Input: part model. Units: mm. Frame: model coordinates. Face numbers are marked on the shaded views. A direction names the side the tool comes from. Round coordinates to 2 decimals unless told otherwise and drop trailing zeros. Loops run counter-clockwise (first coordinate to the right, second up) from the corner with the lowest first, then second, coordinate; pieces in that order, holes last. Notation, with made-up numbers: (-21.5, 86.5) - (31.5, 86.5) arc R23 ccw to (31.5, 96.5) - close; hole circle Ø7 at (23, -26). An arc over 180 degrees is marked (long way). One line per question, with ' | ' between items. Start each with the question number.
from build123d import *

# Parameters (mm, degrees)
BASPROSKE_W        = 10
BASPROSKE_H        = 8
TOOTHCUT_DEPTH     = 16.099668871
TEETHCUTS_COUNT    = 14
TEETHCUTS_ANGLE    = 334.285714286
BORSKE_R           = 0.4
BORE_DEPTH         = 50.0000508
SKETCH1_R          = 3.5
CUT_EXTRUDE1_DEPTH = 10
SKETCH2_W          = 2
SKETCH2_H          = 2
CUT_EXTRUDE2_DEPTH = 10


with BuildPart() as part:
    # BasProSke → Base-Revolve (revolve)
    with BuildSketch(Plane(origin=(0, 0, 0), x_dir=(1, 0, 0), z_dir=(0, 1, 0)), mode=Mode.PRIVATE) as base_revolve_sk:
        with Locations((5, 4)):
            Rectangle(BASPROSKE_W, BASPROSKE_H)
    revolve(base_revolve_sk.sketch.rotate(Axis((-10, 0, 0), (1, 0, 0)), 180), axis=Axis((-10, 0, 0), (1, 0, 0)))

    # TooCutSke → ToothCut (cut, through all)
    with BuildSketch(Plane(origin=(0, 0, 0), x_dir=(0, 0, -1), z_dir=(1, 0, 0))):
        with BuildLine():
            ThreePointArc((0.540393256, 5.723545765), (0, 5.749), (-0.540393256, 5.723545765))
            ThreePointArc((-0.540393256, 5.723545765), (-0.832220085, 6.912663993), (-1.603550271, 7.863566092))
            ThreePointArc((-1.603550271, 7.863566092), (0, 8.0254), (1.603550271, 7.863566092))
            ThreePointArc((1.603550271, 7.863566092), (0.832220085, 6.912663993), (0.540393256, 5.723545765))
        make_face()
    toothcut = extrude(amount=TOOTHCUT_DEPTH, mode=Mode.SUBTRACT)

    # TeethCuts: ToothCut ×14 about axis
    teethcuts_axis = Axis((-10, 0, 0), (1, 0, 0))
    for i in range(1, TEETHCUTS_COUNT):
        add(toothcut.rotate(teethcuts_axis, i * TEETHCUTS_ANGLE / (TEETHCUTS_COUNT - 1)), mode=Mode.SUBTRACT)

    # BorSke → Bore (cut, symmetric)
    with BuildSketch(Plane(origin=(0, 0, 0), x_dir=(0, 0, -1), z_dir=(1, 0, 0))):
        with Locations(Location((0, 0, 0), (0, 0, 180))):
            Circle(BORSKE_R)
    extrude(amount=BORE_DEPTH, both=True, mode=Mode.SUBTRACT)

    # Sketch1 → Cut-Extrude1 (cut)
    with BuildSketch(Plane(origin=(10, 0, 0), x_dir=(0, 0, -1), z_dir=(1, 0, 0))):
        Circle(SKETCH1_R)
    extrude(amount=-CUT_EXTRUDE1_DEPTH, mode=Mode.SUBTRACT)

    # Sketch2 → Cut-Extrude2 (cut)
    with BuildSketch(Plane(origin=(10, 0, 0), x_dir=(0, 0, -1), z_dir=(1, 0, 0))):
        with Locations((0, 3.5)):
            Rectangle(SKETCH2_W, SKETCH2_H)
    extrude(amount=-CUT_EXTRUDE2_DEPTH, mode=Mode.SUBTRACT)


solid = part.part
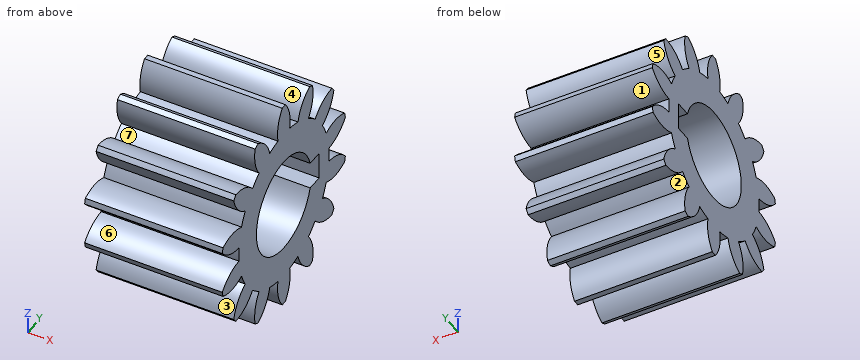
(1) Line query: line 1 along Y through (x, z) = (7.25, 0); line 2 along Z through (x, y) = (6, 0); line 3 along Y through (x, z) = (1, 4.75). Output: solid intervals per line, ascending. Write a range as from..to.
(2) Section A-A, the plane z = 0. Output: boundary loops of the cut face in (x, y), plus the area to 3 significant figures.
(3) Section C-C, the plane z = -6.5. Output: boundary loops of the cut face in (x, y), plus the area to 3 significant figures.
(4) Pin query (flat end, axial travel): P1, Ø0.9, axis at x = 4.5, y = 4, coming from the -Z side; P2, Ø3, axis at x = 2.5, z = -4.5, coming from the -Y side; P3, Ø2, axis at x = 8, y = 1.5, coming from the -Z side; P4, Ø5.5, axis at y = 0, z = 0, coming from the -X side. Return the tip coordinate at first contact, or that it passes through.
(5) Reachability of the marked faces 1, 2, 3 and 4 from +Z, -Z, +X, -X, +Y, -Y: full face, straight path, thin tool, end or side. Return the list, or none.
(6) Section B-B, the plane y = 0. Output: boundary loops of the cut face in (x, z), plus the area to 3 significant figures.
(7) Pull-direction query (Y, two-part tool) for the marked faces 5, 6 and 7; classes: released by +Y, released by -Y, zero draft, split by the parting line, or undercut.
Derived:
1) line 1: y = -5.75..-3.5, 4.5..5.75 | line 2: z = -8..-3.5, 3.5..8 | line 3: y = -6.36..-4.71, -3.24..3.24, 4.71..6.36
2) outline: (0, -5.75) - (10, -5.75) - (10, -3.5) - (0, -3.5) - close; (0, 4.5) - (10, 4.5) - (10, 5.75) - (0, 5.75) - close | area: 35.0 mm²
3) outline: (0, -3.72) - (10, -3.72) - (10, -2.31) - (0, -2.31) - close; (0, -0.8) - (10, -0.8) - (10, 0.8) - (0, 0.8) - close; (0, 2.31) - (10, 2.31) - (10, 3.72) - (0, 3.72) - close | area: 44.2 mm²
4) P1: stops at z = -7.17 | P2: stops at y = -6.38 | P3: stops at z = -7.54 | P4: passes through
5) face 1: +X, -X, +Y | face 2: +X, -X | face 3: +X, -X, -Y | face 4: +Z, +X, -X
6) outline: (0, -8) - (10, -8) - (10, -3.5) - (0, -3.5) - close; (0, 3.5) - (10, 3.5) - (10, 8) - (0, 8) - close | area: 90.0 mm²
7) face 5: released by +Y | face 6: released by -Y | face 7: undercut
